Autodesk Inventor part; units mm, degrees
ref_plane "Pracovní rovina1" through (0, 12.5, 0) normal (0, -1, 0) x (1, 0, 0)
ref_plane "YZ Plane" through (0, 0, 0) normal (1, 0, 0) x (0, 1, 0)
ref_plane "XZ Plane" through (0, 0, 0) normal (0, 1, 0) x (-1, 0, 0)
sketch "Náčrt1" plane through (0, 0, 0) normal (0, 0, 1) x (1, 0, 0)
  circle A0 centre (0, 0) radius 14
  dimension "d0" = 28
extrude "Vysunutí1" add sketch "Náčrt1" along normal mid plane 25
sketch "Náčrt2" plane through (0, 0, 0) normal (1, 0, 0) x (0, 1, 0)
  line L0 (-14, -12.5) -> (14, -12.5)
  line L1 (14, 12.5) -> (-14, 12.5)
  line L2 (14, -12.5) -> (14, 12.5)
  line L3 (14, 11) -> (12.5, 11)
  line L4 (12.5, 11) -> (12.5, -11)
  line L5 (12.5, -11) -> (14, -11)
  line L6 (14, -11) -> (14, 11)
  line L7 (14, 0) -> (-14, 0) construction
  line L8 (-14, -12.5) -> (-14, 12.5)
  line L9 (0, 12.5) -> (0, -12.5) construction
  point P0 (0, 0)
  point P1 (14, -11)
  dimension "d4" = 11
  dimension "d5" = 12.5
revolve "Rotace1" cut sketch "Náčrt2" angle 360 about axis through (0, 0, 12.5) along (0, 0, -1) contours L5 L4 L3 L2
sketch "Náčrt3" plane through (0, 0, -12.5) normal (0, 0, -1) x (-1, 0, 0)
  line L0 (-6, 5) -> (6, 5)
  line L1 (6, 5) -> (6, -5)
  line L2 (6, -5) -> (-6, -5)
  line L3 (-6, -5) -> (-6, 5)
  line L4 (-6, 5) -> (6, -5) construction
  line L5 (6, 5) -> (-6, -5) construction
  circle A0 centre (0, 0) radius 9
  dimension "d7" = 12
  dimension "d8" = 10
  dimension "d9" = 18
hole "Díra1" at (0, 0, -12.5) direction (0, 0, 1) diameter 18 depth 10
sketch "Náčrt4" plane through (0, 0, 12.5) normal (0, 0, 1) x (1, 0, 0)
  circle A0 centre (0, 0) radius 14
hole "Díra2" at (0, 0, 12.5) direction (0, 0, -1) diameter 3 end through all
ref_plane "Pracovní rovina1" through (0, 12.5, 0) normal (0, -1, 0) x (1, 0, 0)
sketch "Náčrt5" plane through (0, 12.5, 0) normal (0, -1, 0) x (1, 0, 0)
  line L0 (1.5, -2.5) -> (-1.5, -2.5)
  line L1 (-9, -2.5) -> (9, -2.5)
  line L2 (0, 0) -> (0, -10.7479) construction
  point P0 (0, 1.5)
  point P1 (0, 5.5)
  dimension "d24" = 4
  dimension "d25" = 4
hole "Díra3" at (0, 12.5, 1.5) at (0, 12.5, 5.5) direction (0, -1, 0) diameter 3 depth 12.5
thread "Závit1"
thread "Závit2"
chamfer "Zkosení1" distance 1 angle 45 1 edges at (0, -9, -12.5)
fillet "Zaoblení1" radius 1 1 edges at (0, -9, -2.5)
properties part number "Wheel"
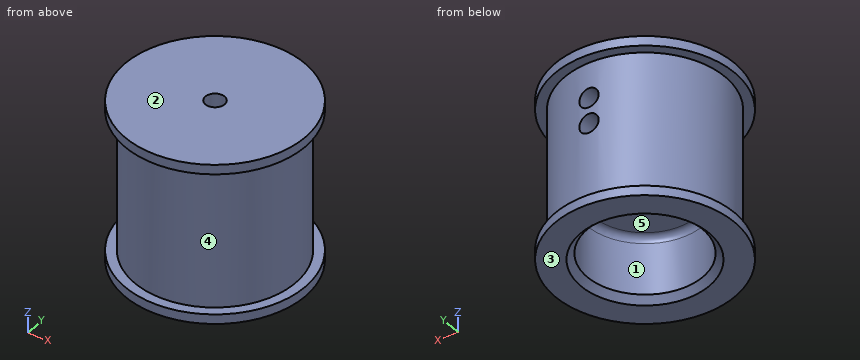
Here's how the part is built. I have some questions about the finished solid (model axes, mm). Face numbers are marked on the shaded views. A direction names the side the tool comes from. Give positions to 0.01 mm unless a question says otherwise; leave off trailing zeros. Order: outer loops, then holes, each group sorted by start corner. A loop starts at its lowest first (then second) coordinate and runs counter-clockwise, first axis right, second up. Notation, with made-up numbers: M -29.75,36.25 L -4.75,36.25 A32 cw -4.75,68.25 Z; hole C 0,-35 d10. An arc over 180 degrees is marked long. Use a Markdown table: item, result. Add a question column.
1. Suppose I cut it at B-B (z = 8). List the corners of the cut face in (x, y) for me.
2. If we mould it in two halves opening along Y, with no side actions, what happens to the marked faces 3, 4 and 5? For each: +Y half, -Y half, draft (parallel to the pull), parting line (faces both ways), or undercut.
3. For pin 1 Ø3 at (x, z) = (0.5, -3) entering from -Y; pin 2 Ø1.8 at (x, z) = (0, 5.5) entering from +Y; pin 3 Ø8 at (y, z) = (6.5, -3) entering from -X, each with a flat end and sliding along its axis, tell me the tip position at first contact or that it passes through.
4. Suppose I cut it at D-D (x = -11.25). List the corners of the cut face in (y, z) for me.
5. I need wall thicknesses on probe 1 along X at (y, z) = (0, 9.5); probe 2 along X at (y, z) = (0, -9); probe 3 along Z at (x, y) = (0.5, 8). Which ranges of each line are inside material? Lowest first, please. Write a range as from..to.
6. Suppose I cut it at A-A (x = 0). Give the number of separate pieces and of enclosed holes in the cut face, and give its area (3 significant figures).
7. On a 3-axis mill with a long thin cutter (end or side, diameter ignored), from which of +Z, -Z, +X, -X, +Y, -Y can I reach the whole of each face in a straight line? I mean the marked faces 1 and 2. Say none if no direction works.
Results list:
| question | item | result |
|---|---|---|
| 1 | outline | C 0,0 d25; hole C 0,0 d3 |
| 2 | face 3 | draft |
| 2 | face 4 | parting line |
| 2 | face 5 | undercut |
| 3 | pin 1 | stops at y = -12.5 |
| 3 | pin 2 | stops at y = -1.2 |
| 3 | pin 3 | stops at x = -12.25 |
| 4 | outline | M -8.33,-12.5 L 8.33,-12.5 L 8.33,-11 L 5.45,-11 L 5.45,11 L 8.33,11 L 8.33,12.5 L -8.33,12.5 L -8.33,11 L -5.45,11 L -5.45,-11 L -8.33,-11 Z |
| 5 | probe 1 | x = -12.5..-1.5, 1.5..12.5 |
| 5 | probe 2 | x = -12.5..-9, 9..12.5 |
| 5 | probe 3 | z = -2.5..0.09, 2.91..4.09, 6.91..12.5 |
| 6 | separate pieces | 4 |
| 6 | enclosed holes | 0 |
| 6 | area | 342 mm² |
| 7 | face 1 | -Z |
| 7 | face 2 | +Z, +X, -X, +Y, -Y |
